Verification items for the finished model (mm, model axes). Coordinates: 2 decimals unless noted, no trailing zeros. Loops run counter-clockwise (first coordinate to the right, second up) from the corner with the lowest first, then second, coordinate; pieces in that order, holes last. Notation, with made-up numbers: (-17, -11) -> (39, -11) arc R23 cw to (39, -2) -> close; hole circle Ø10 at (87.5, 73.5). An arc over 180 degrees is marked (long way). Answer as a JSON object with one key per item and string values. Group by question number.
Q1. Cross-section at A-A on y = 143. Record the boundary of the cut face in (x, z).
Q2. Cross-section at C-C on x = 722. Record the boundary of the cut face in (y, z), and give its area (3 significant figures).
Q3. Scan lines: L1, parallel to Y at x = 691, z = 0.45; L2, parallel to X at y = 121.5, z = 1.6; L3, parallel to X at y = 126.5, z = 1.1. Record each from-to range of solid material in increasing order.
Q4. Cross-section at B-B on x = 698. Record the boundary of the cut face in (y, z).
Q5. Gauge pin test, flat ends, axial feed: pin 1 Ø1 at (y, z) = (108, 1.5) entering from -X; pin 2 Ø0.6 at (y, z) = (114.5, 1) entering from +X; pin 3 Ø1 at (x, z) = (704, 1.5) entering from +Y. Record the tip position at first contact, or that the pin passes through.
```python
from build123d import *

# Parameters (mm, degrees)
EXTRUDE_1_DEPTH = 2


with BuildPart() as part:
    # Model → 凸台-拉伸1 (new body)
    with BuildSketch(Plane.XY):
        Polygon((682.151439572, 151.342718787), (685.151439572, 151.342718787), (685.151439572, 154.342718787), (690.151439572, 154.342718787), (690.151439572, 157.342718787), (700.151439572, 157.342718787), (700.151439572, 154.342718787), (705.151439572, 154.342718787), (705.151439572, 157.342718787), (715.151439572, 157.342718787), (715.151439572, 154.342718787), (720.151439572, 154.342718787), (720.151439572, 151.342718787), (723.151439572, 151.342718787), (725.151439572, 151.342718787), (725.151439572, 145.282718787), (726.651439572, 145.282718787), (726.651439572, 135.282718787), (725.151439572, 135.282718787), (725.151439572, 130.072718787), (725.151439572, 125.282718787), (726.651439572, 125.282718787), (726.651439572, 115.282718787), (725.151439572, 115.282718787), (725.151439572, 111.972718787), (720.151439572, 111.972718787), (720.151439572, 108.972718787), (715.151439572, 108.972718787), (715.151439572, 105.972718787), (705.151439572, 105.972718787), (705.151439572, 108.972718787), (700.151439572, 108.972718787), (700.151439572, 105.972718787), (690.151439572, 105.972718787), (690.151439572, 108.972718787), (685.151439572, 108.972718787), (685.151439572, 111.972718787), (680.151439572, 111.972718787), (680.151439572, 115.282718787), (678.651439572, 115.282718787), (678.651439572, 125.282718787), (680.151439572, 125.282718787), (680.151439572, 130.072718787), (680.151439572, 135.282718787), (678.651439572, 135.282718787), (678.651439572, 145.282718787), (680.151439572, 145.282718787), (680.151439572, 151.342718787), align=None)
        with BuildLine():
            Line((714.151439572, 148.342718787), (691.151439572, 148.342718787))
            ThreePointArc((691.151439572, 148.342718787), (689.030119228, 147.46403913), (688.151439572, 145.342718787))
            Line((688.151439572, 145.342718787), (688.151439572, 117.972718787))
            ThreePointArc((688.151439572, 117.972718787), (689.030119228, 115.851398443), (691.151439572, 114.972718787))
            Line((691.151439572, 114.972718787), (714.151439572, 114.972718787))
            ThreePointArc((714.151439572, 114.972718787), (716.272759915, 115.851398443), (717.151439572, 117.972718787))
            Line((717.151439572, 117.972718787), (717.151439572, 145.342718787))
            ThreePointArc((717.151439572, 145.342718787), (716.272759915, 147.46403913), (714.151439572, 148.342718787))
        make_face(mode=Mode.SUBTRACT)
    extrude(amount=EXTRUDE_1_DEPTH)


solid = part.part
```
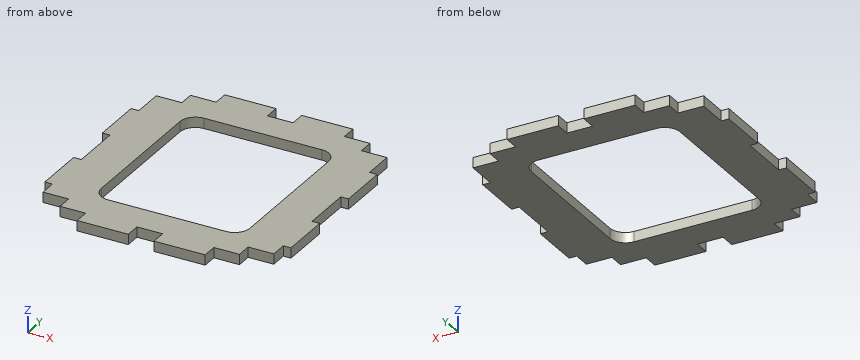
Computed values:
{
 "1": {"outline": "(678.65, 0) -> (688.15, 0) -> (688.15, 2) -> (678.65, 2) -> close; (717.15, 0) -> (726.65, 0) -> (726.65, 2) -> (717.15, 2) -> close"},
 "2": {"outline": "(111.97, 0) -> (151.34, 0) -> (151.34, 2) -> (111.97, 2) -> close", "area": "78.7 mm²"},
 "3": {"L1": "y = 105.97 to 114.98, 148.34 to 157.34", "L2": "x = 678.65 to 688.15, 717.15 to 726.65", "L3": "x = 680.15 to 688.15, 717.15 to 725.15"},
 "4": {"outline": "(105.97, 0) -> (114.97, 0) -> (114.97, 2) -> (105.97, 2) -> close; (148.34, 0) -> (157.34, 0) -> (157.34, 2) -> (148.34, 2) -> close"},
 "5": {"pin 1": "stops at x = 690.15", "pin 2": "stops at x = 725.15", "pin 3": "stops at y = 154.34"}
}
